Geometry check sheet. Reference: the model listing, model coordinates, mm. Coordinates: 2 decimals unless noted, no trailing zeros. Loops run counter-clockwise (first coordinate to the right, second up) from the corner with the lowest first, then second, coordinate; pieces in that order, holes last.
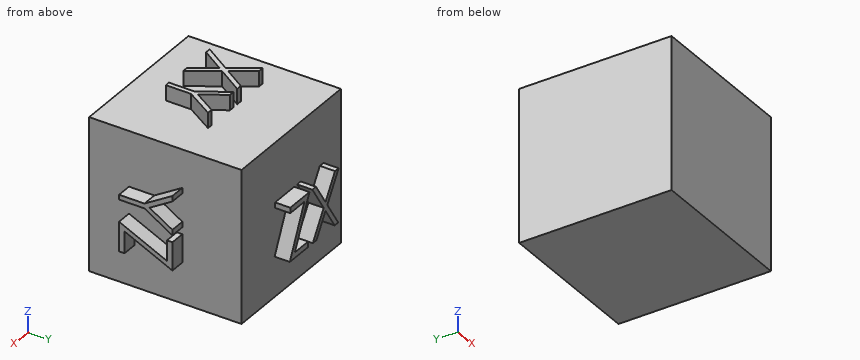
from build123d import *

# Parameters (mm, degrees)
SKETCH1_W           = 10
SKETCH1_H           = 10
BOSS_EXTRUDE1_DEPTH = 10
BOSS_EXTRUDE2_DEPTH = 1
BOSS_EXTRUDE3_DEPTH = 1
BOSS_EXTRUDE4_DEPTH = 1


with BuildPart() as part:
    # Sketch1 → Boss-Extrude1 (new body)
    with BuildSketch(Plane(origin=(0, 0, 0), x_dir=(1, 0, 0), z_dir=(0, 1, 0))):
        with Locations((5, 5)):
            Rectangle(SKETCH1_W, SKETCH1_H)
    extrude(amount=BOSS_EXTRUDE1_DEPTH)

    # Sketch2 → Boss-Extrude2 (add)
    with BuildSketch(Plane.XY):
        Polygon((1.888096604, 6.09581066), (2.250576572, 6.09581066), (3.166942757, 4.664119955), (4.083308943, 6.09581066), (4.445788911, 6.09581066), (3.348533302, 4.38086675), (4.490660706, 2.59581066), (4.128180738, 2.59581066), (3.166942757, 4.097613545), (2.205704777, 2.59581066), (1.843224809, 2.59581066), (2.986053334, 4.38086675), align=None)
        Polygon((4.827199168, 6.09581066), (5.186874649, 6.09581066), (6.106746443, 4.59190441), (7.025215995, 6.09581066), (7.384891475, 6.09581066), (6.263096604, 4.25957268), (6.263096604, 2.59581066), (5.94899404, 2.59581066), (5.94899404, 4.25957268), align=None)
    extrude(amount=BOSS_EXTRUDE2_DEPTH)

    # Sketch3 → Boss-Extrude3 (add)
    with BuildSketch(Plane(origin=(0, 10, 0), x_dir=(1, 0, 0), z_dir=(0, 1, 0))):
        Polygon((1.802209363, 7.38229402), (2.164689331, 7.38229402), (3.081055517, 5.950603315), (3.997421703, 7.38229402), (4.359901671, 7.38229402), (3.262646062, 5.667350109), (4.404773466, 3.88229402), (4.042293498, 3.88229402), (3.081055517, 5.384096904), (2.119817536, 3.88229402), (1.757337568, 3.88229402), (2.900166094, 5.667350109), align=None)
        Polygon((4.831055517, 7.023319661), (4.831055517, 7.38229402), (6.670799107, 7.38229402), (5.202650068, 4.241268379), (6.625927312, 4.241268379), (6.625927312, 3.88229402), (4.696440132, 3.88229402), (6.164589171, 7.023319661), align=None)
    extrude(amount=BOSS_EXTRUDE3_DEPTH)

    # Sketch4 → Boss-Extrude4 (add)
    with BuildSketch(Plane(origin=(10, 0, 0), x_dir=(0, 0, -1), z_dir=(1, 0, 0))):
        Polygon((2.493902055, 6.115757789), (2.853577536, 6.115757789), (3.773449331, 4.611851539), (4.691918882, 6.115757789), (5.051594363, 6.115757789), (3.929799491, 4.279519808), (3.929799491, 2.615757789), (3.615696927, 2.615757789), (3.615696927, 4.279519808), align=None)
        Polygon((5.500312311, 5.75678343), (5.500312311, 6.115757789), (7.340055901, 6.115757789), (5.871906863, 2.974732148), (7.295184106, 2.974732148), (7.295184106, 2.615757789), (5.365696927, 2.615757789), (6.833845965, 5.75678343), align=None)
    extrude(amount=BOSS_EXTRUDE4_DEPTH)


solid = part.part
1) Depth check by flat-ended pin: pin 1 (0.8 mm diameter, centred on x = 10.5, z = -6.5, fed in from -Y). Enter the tip coordinate at first touch or a pass-through.
Data:
pin 1: stops at y = 2.62
2) Section check C-C on z = -6.5. Record the cut outline in (x, y), and give its area (3 significant figures).
Data:
outline: (0, 0) - (10, 0) - (10, 2.62) - (11, 2.62) - (11, 2.97) - (10, 2.97) - (10, 4.32) - (11, 4.32) - (11, 5.04) - (10, 5.04) - (10, 5.76) - (11, 5.76) - (11, 6.12) - (10, 6.12) - (10, 10) - (6.26, 10) - (6.26, 11) - (5.92, 11) - (5.92, 10) - (3.8, 10) - (3.8, 11) - (3.43, 11) - (3.43, 10) - (2.73, 10) - (2.73, 11) - (2.37, 11) - (2.37, 10) - (0, 10) - close
area: 103 mm2
3) Section check A-A on z = 0.25. Record the cut outline in (x, y), and give its area (3 significant figures).
Data:
outline: (1.84, 2.6) - (2.21, 2.6) - (3.17, 4.1) - (4.13, 2.6) - (4.49, 2.6) - (3.35, 4.38) - (4.45, 6.1) - (4.08, 6.1) - (3.17, 4.66) - (2.25, 6.1) - (1.89, 6.1) - (2.99, 4.38) - close; (4.83, 6.1) - (5.95, 4.26) - (5.95, 2.6) - (6.26, 2.6) - (6.26, 4.26) - (7.38, 6.1) - (7.03, 6.1) - (6.11, 4.59) - (5.19, 6.1) - close
area: 4.21 mm2
4) Section check D-D on x = 8.5. Record the cut outline in (y, z), and give its area (3 significant figures).
Data:
outline: (0, -10) - (10, -10) - (10, 0) - (0, 0) - close
area: 100 mm2
5) Material ranges on probe 1 along Z at (x, y) = (5.5, 10.75); probe 2 along Y at (x, z) = (1, -8); probe 3 along Z at (x, y) = (4, 4), recorded low to high.
Data:
probe 1: z = -7.38 to -7.02, -5.6 to -4.88, -4.24 to -3.88
probe 2: y = 0 to 10
probe 3: z = -10 to 0
